Part model, mm, in its own coordinate system. Face numbers are marked on the shaded views. Give positions to 0.01 mm unless a question says otherwise; leave off trailing zeros. Write each loop counter-clockwise with the first axis right and the second up, starting at its lowest first coordinate (ties: lowest second). Pieces come first, ordered by that corner, then holes.
Autodesk Inventor part; units mm, degrees
ref_plane "YZ Plane" through (0, 0, 0) normal (1, 0, 0) x (0, 1, 0)
ref_plane "XZ Plane" through (0, 0, 0) normal (0, 1, 0) x (-1, 0, 0)
ref_plane "XY Plane" through (0, 0, 0) normal (0, 0, 1) x (1, 0, 0)
sketch "Sketch1" plane through (0, 0, 0) normal (0, 0, 1) x (1, 0, 0)
  line L0 (0, 0) -> (-80, 0)
  line L1 (-80, 0) -> (-80, 80)
  line L2 (-80, 80) -> (0, 80)
  line L3 (0, 80) -> (0, 0)
  line L4 (-75, 75) -> (-5, 75)
  line L5 (-5, 75) -> (-5, 5)
  line L6 (-5, 5) -> (-75, 5)
  line L7 (-75, 5) -> (-75, 75)
  dimension "d0" = 80
  dimension "d1" = 80
  dimension "d2" = 70
  dimension "d3" = 70
extrude "Extrusion1" add sketch "Sketch1" along normal blind 7 contours L0 L1 L2 L3 | L4 L5 L6 L7
sketch "Sketch2" plane through (-80, 80, 0) normal (0, 1, 0) x (1, 0, 0)
  line L0 (24.4, -3.45) -> (15.6, -3.45)
  line L1 (15.6, -3.45) -> (15.6, -6.55)
  line L2 (15.6, -6.55) -> (24.4, -6.55)
  line L3 (24.4, -6.55) -> (24.4, -3.45)
  line L4 (64.4, -3.45) -> (55.6, -3.45)
  line L5 (55.6, -3.45) -> (55.6, -6.55)
  line L6 (55.6, -6.55) -> (64.4, -6.55)
  line L7 (64.4, -6.55) -> (64.4, -3.45)
  point P0 (80, 0)
  point P1 (20, -5)
  point P2 (60, -5)
  dimension "d8" = 8.8
  dimension "d9" = 3.1
  dimension "d12" = 8.8
  dimension "d13" = 3.1
extrude "Extrusion2" [suppressed]
sketch "Sketch4" plane through (0, 0, 7) normal (0, 0, 1) x (1, 0, 0)
  line L0 (-5, 5) -> (-75, 5)
  line L1 (-75, 5) -> (-75, 75)
  line L2 (-75, 75) -> (-5, 75)
  line L3 (-5, 75) -> (-5, 5)
  point P0 (0, 0)
  point P1 (-7.5, 40)
  point P2 (-72.5, 40)
  dimension "d21" = 70
  dimension "d22" = 70
extrude "Extrusion3" cut sketch "Sketch4" against normal blind 4
sketch "Sketch5" plane through (-80, 0, 0) normal (0, -1, 0) x (1, 0, 0)
  line L0 (2, 2) -> (12, 2)
  line L1 (12, 2) -> (12, 5)
  line L2 (12, 5) -> (2, 5)
  line L3 (2, 5) -> (2, 2)
  line L4 (78, 2) -> (68, 2)
  line L5 (68, 2) -> (68, 5)
  line L6 (68, 5) -> (78, 5)
  line L7 (78, 5) -> (78, 2)
  point P0 (80, 0)
  dimension "d25" = 10
  dimension "d26" = 3
  dimension "d27" = 10
  dimension "d28" = 3
extrude "Extrusion4" [suppressed]
sketch "Sketch8" plane through (0, 0, 7) normal (0, 0, 1) x (1, 0, 0)
  circle A0 centre (-7.5, 40) radius 3
  circle A1 centre (-72.5, 40) radius 4
  point P0 (0, 0)
  dimension "d42" = 6
  dimension "d43" = 8
extrude "Extrusion5" cut sketch "Sketch8" against normal blind 4
sketch "Sketch9" plane through (0, 0, 3) normal (0, 0, 1) x (1, 0, 0)
  point P0 (0, 0)
  point P1 (-7.5, 40)
  point P2 (-72.5, 40)
hole "Hole2" at (-7.5, 40, 3) at (-72.5, 40, 3) direction (0, 0, -1) diameter 4 depth 8
sketch "Sketch11" plane through (0, 0, 3) normal (0, 0, 1) x (1, 0, 0)
  line L0 (-5, 38.3417) -> (-5, 5)
  line L1 (-5, 5) -> (-75, 5)
  line L2 (-75, 5) -> (-75, 35)
  line L3 (-75, 35) -> (-5, 35)
  line L4 (-5, 35) -> (-5, 5)
  line L5 (-75, 43.1225) -> (-75, 75)
  line L6 (-75, 75) -> (-5, 75)
  line L7 (-5, 75) -> (-5, 45)
  line L8 (-5, 45) -> (-75, 45)
  line L9 (-75, 45) -> (-75, 75)
  line L10 (-65, 35) -> (-15, 35)
  line L11 (-15, 35) -> (-15, 45)
  line L12 (-15, 45) -> (-65, 45)
  line L13 (-65, 45) -> (-65, 35)
  point P0 (0, 0)
  dimension "d60" = 70
  dimension "d61" = 30
  dimension "d62" = 70
  dimension "d63" = 30
  dimension "d66" = 50
extrude "Extrusion7" add sketch "Sketch11" along normal blind 2
properties part number "Marker_TestFit"
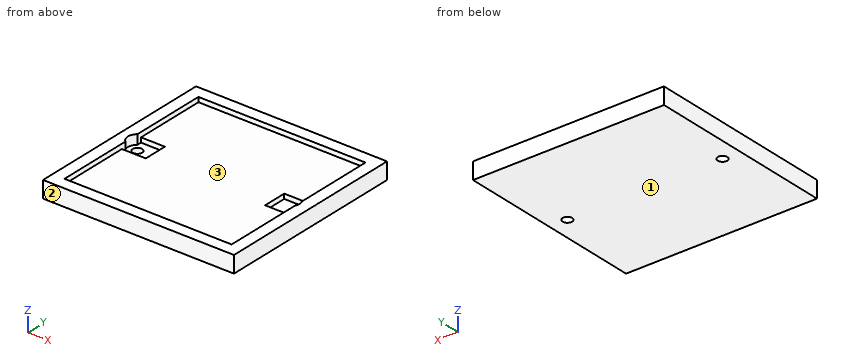
1) Saw through at C-C (z = 4). Write the cut outline in (x, y), and give its area (3 significant figures).
Check result:
outline: (-80, 0) - (0, 0) - (0, 80) - (-80, 80) - close; hole (-75, 35) - (-65, 35) - (-65, 45) - (-75, 45) - (-75, 43.12) arc R4 ccw to (-75, 36.88) - close; hole (-15, 35) - (-5, 35) - (-5, 38.34) arc R3 ccw to (-5, 41.66) - (-5, 45) - (-15, 45) - close
area: 6,190 mm2
2) Saw through at A-A (y = 40). Write the cut outline in (x, z), and give its area (3 significant figures).
Check result:
outline: (-80, 0) - (-74.5, 0) - (-74.5, 3) - (-76.5, 3) - (-76.5, 7) - (-80, 7) - close; (-70.5, 0) - (-9.5, 0) - (-9.5, 3) - (-15, 3) - (-15, 5) - (-65, 5) - (-65, 3) - (-70.5, 3) - close; (-5.5, 0) - (0, 0) - (0, 7) - (-4.5, 7) - (-4.5, 3) - (-5.5, 3) - close
area: 348 mm2
3) Saw through at D-D (y = 29). Write the cut outline in (x, z), and give its area (3 significant figures).
Check result:
outline: (-80, 0) - (0, 0) - (0, 7) - (-5, 7) - (-5, 5) - (-75, 5) - (-75, 7) - (-80, 7) - close
area: 420 mm2
4) Saw through at B-B (x = -7.5). Write the cut outline in (y, z).
Check result:
outline: (0, 0) - (38, 0) - (38, 3) - (35, 3) - (35, 5) - (5, 5) - (5, 7) - (0, 7) - close; (42, 0) - (80, 0) - (80, 7) - (75, 7) - (75, 5) - (45, 5) - (45, 3) - (42, 3) - close
5) Mould opens along Y. For the marked faces 1, 2 and 3 say: +Y half, -Y half, draft (parallel to the pull), parting line (faces both ways), or undercut.
Check result:
face 1: draft
face 2: -Y half
face 3: undercut
6) Drill centre lines: L1, parallel to X at y = 40, z = 1.2; L2, parallel to Y at x = -44, z = 6.25; L3, parallel to X at y = 23, z = 5.25. Where is each one in solid material? Low to high.
Check result:
L1: x = -80 to -74.5, -70.5 to -9.5, -5.5 to 0
L2: y = 0 to 5, 75 to 80
L3: x = -80 to -75, -5 to 0
7) Flat gauge pins, fed straight in: P1, Ø5, axis at x = -7.5, y = 40, coming from the +Z side; P2, Ø8, axis at x = -29.5, y = 46.5, coming from the +Z side. Where does each tip first touch, or does it go through?
Check result:
P1: stops at z = 3
P2: stops at z = 5
